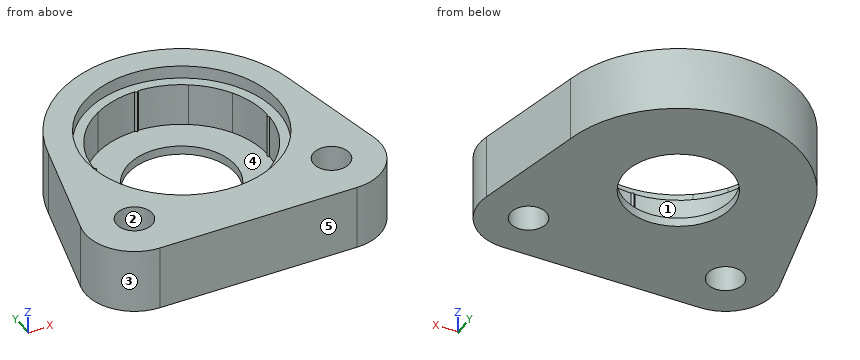
Autodesk Inventor part; units mm, degrees
ref_plane "YZ Plane" through (0, 0, 0) normal (1, 0, 0) x (0, 1, 0)
ref_plane "XZ Plane" through (0, 0, 0) normal (0, 1, 0) x (-1, 0, 0)
ref_plane "XY Plane" through (0, 0, 0) normal (0, 0, 1) x (1, 0, 0)
sketch "Sketch1" plane through (0, 0, 0) normal (0, 0, 1) x (1, 0, 0)
  arc A0 (-5.827627, -9.579088) -> (-0.250527, -11.231057) centre (0.025157, -0.060123) ccw
  arc A1 (0.25, -11.209713) -> (5.829601, -9.582326) centre (0.025157, -0.060123) ccw
  line L0 (0.46552, -11.403002) -> (0, -10.9855)
  line L1 (0, -10.9855) -> (-0.46552, -11.403002)
  arc A2 (-11.176173, -0.249433) -> (-9.579088, -5.827627) centre (0.025157, -0.060123) ccw
  line L2 (-11.403002, -0.46552) -> (-10.9855, 0)
  line L3 (-10.9855, 0) -> (-11.403002, 0.46552)
  arc A3 (-9.579088, 5.827627) -> (-11.209713, 0.25) centre (0, 0) ccw
  arc A4 (5.827627, 9.579088) -> (0.25, 11.209713) centre (0, 0) ccw
  line L4 (0, 10.9855) -> (0.46552, 11.403002)
  line L5 (-0.46552, 11.403002) -> (0, 10.9855)
  arc A5 (-0.25, 11.209713) -> (-5.827627, 9.579088) centre (0, 0) ccw
  arc A6 (11.209713, 0.25) -> (9.579088, 5.827627) centre (0, 0) ccw
  line L6 (11.403002, 0.46552) -> (10.9855, 0)
  line L7 (10.9855, 0) -> (11.403002, -0.46552)
  arc A7 (9.579088, -5.827627) -> (11.209713, -0.25) centre (0, 0) ccw
  arc A8 (7.230816, -10.196338) -> (10.196338, -7.230816) centre (0, 0) ccw
  arc A9 (-10.196338, -7.230816) -> (-7.230816, -10.196338) centre (0, 0) ccw
  arc A10 (-7.230816, 10.196338) -> (-10.196338, 7.230816) centre (0, 0) ccw
  circle A11 centre (0, 0) radius 12.5
  circle A12 centre (12.7, -12.7) radius 2.3241
  circle A13 centre (-12.7, -12.7) radius 2.3241
  line L8 (-19.05, -12.7) -> (19.05, -12.7) construction
  line L9 (-12.7, -19.05) -> (12.7, -19.05)
  line L10 (12.7, -6.35) -> (-12.7, -6.35)
  arc A14 (-12.7, -6.35) -> (-12.7, -19.05) centre (-12.7, -12.7) ccw
  arc A15 (12.7, -19.05) -> (12.7, -6.35) centre (12.7, -12.7) ccw
  circle A16 centre (0, 0) radius 11.2125
  circle A17 centre (0, 0) radius 15.875
  line L11 (15.560093, 3.146287) -> (18.887388, -11.272158)
  line L12 (0, -10.9855) -> (0, -12.5)
  line L13 (-15.560093, 3.146287) -> (-18.887388, -11.272158)
  point P0 (-0.46552, -11.403002)
  point P1 (-11.403002, -0.46552)
  point P2 (0, -12.7)
  point P3 (10.196338, -7.230816)
  point P4 (7.230816, -10.196338)
  point P5 (-7.230816, -10.196338)
  point P6 (-10.196338, -7.230816)
  point P7 (-10.196338, 7.230816)
  point P8 (-7.230816, 10.196338)
  point P9 (-0.25, -11.209713)
  point P10 (0.25, -11.209713)
  point P11 (9.579088, -5.827627)
  point P12 (9.579088, 5.827627)
  point P13 (-5.827627, 9.579088)
  point P14 (-9.579088, 5.827627)
  point P15 (-11.209713, -0.25)
  dimension "d0" = 25
  dimension "d9" = 31.75
  dimension "d1" = 4.6482
  dimension "d2" = 4.6482
  dimension "d4" = 6.35
  dimension "d5" = 6.35
  dimension "d6" = 12.7
  dimension "d8" = 25.4
extrude "Extrusion1" add sketch "Sketch1" along normal blind 12.7 contours L10 A14 A17 A15 A11 A10 | A11 A9 A8 L10 A15 A17 A12 A13 A14 | A17 A13 A12 A15 L9 A14 | A14 L13 A17 | A17 L11 A15
extrude "Extrusion2" add sketch "Sketch1" along normal blind 10.9982 contours A16 L1 A0 | A0 L1 A16 L12 A11 A9 L10 | A16 L10 L0 L1 | A16 L2 L3 A3 A5 L5 L4 A4 A6 L6 L7 A7 L10 | L10 A11 A10 A16 A7 A6 A4 A5 A3 | L1 L12 A16 | L10 A11 A8 L12 A16 | L0 A16 L12 | A16 L3 L2 | L7 L6 A16 | A16 L4 L5
sketch "Sketch1 outline for Extrusion3" plane through (0, 0, 0) normal (0, 0, 1) x (1, 0, 0)
  arc A0 (-11.209713, -0.25) -> (-0.25, -11.209713) centre (0, 0) ccw
  line L0 (-10.9855, 0) -> (-11.209713, -0.25)
  line L1 (-11.209713, 0.25) -> (-10.9855, 0)
  arc A1 (-9.579088, 5.827627) -> (-11.209713, 0.25) centre (0, 0) ccw
  arc A2 (-5.827627, 9.579088) -> (-9.579088, 5.827627) centre (0, 0) ccw
  arc A3 (-0.25, 11.209713) -> (-5.827627, 9.579088) centre (0, 0) ccw
  line L2 (0, 10.9855) -> (-0.25, 11.209713)
  line L3 (0.25, 11.209713) -> (0, 10.9855)
  arc A4 (5.827627, 9.579088) -> (0.25, 11.209713) centre (0, 0) ccw
  arc A5 (9.579088, 5.827627) -> (5.827627, 9.579088) centre (0, 0) ccw
  arc A6 (11.209713, 0.25) -> (9.579088, 5.827627) centre (0, 0) ccw
  line L4 (10.9855, 0) -> (11.209713, 0.25)
  line L5 (11.209713, -0.25) -> (10.9855, 0)
  arc A7 (9.579088, -5.827627) -> (11.209713, -0.25) centre (0, 0) ccw
  arc A8 (0.25, -11.209713) -> (9.579088, -5.827627) centre (0, 0) ccw
  line L6 (0, -10.9855) -> (0.25, -11.209713)
  line L7 (-0.25, -11.209713) -> (0, -10.9855)
extrude "Extrusion3" cut sketch "Sketch1 outline for Extrusion3" along normal blind 10.9982
sketch "Sketch2" plane through (0, 0, 0) normal (0, 0, -1) x (-1, 0, 0)
  arc A0 (-0.25, 11.209713) -> (-11.209713, 0.25) centre (0, 0) ccw
  arc A1 (11.209713, 0.25) -> (0.25, 11.209713) centre (0, 0) ccw
  line L0 (0, 10.9855) -> (0.25, 11.209713)
  line L1 (-0.25, 11.209713) -> (0, 10.9855)
  line L2 (11.209713, 0.25) -> (10.9855, 0)
  line L3 (10.9855, 0) -> (11.209713, -0.25)
  arc A2 (0.25, -11.209713) -> (11.209713, -0.25) centre (0, 0) ccw
  line L4 (0.25, -11.209713) -> (0, -10.9855)
  line L5 (0, -10.9855) -> (-0.25, -11.209713)
  arc A3 (-11.209713, -0.25) -> (-0.25, -11.209713) centre (0, 0) ccw
  line L6 (-11.209713, -0.25) -> (-10.9855, 0)
  line L7 (-10.9855, 0) -> (-11.209713, 0.25)
  circle A4 centre (0, 0) radius 6.9977
  point P0 (0, 0)
  dimension "d16" = 13.9954
extrude "Extrusion4" add sketch "Sketch2" against normal blind 5.3848
sketch "Sketch3" plane through (0, 0, 0) normal (0, 0, -1) x (-1, 0, 0)
  circle A0 centre (0, 0) radius 6.9977
  arc A1 (12.7, -19.05) -> (18.887388, -11.272158) centre (12.7, -12.7) ccw
  line L0 (15.560093, 3.146287) -> (18.887388, -11.272158)
  arc A2 (15.560093, 3.146287) -> (-15.560093, 3.146287) centre (0, 0) ccw
  line L1 (-18.887388, -11.272158) -> (-15.560093, 3.146287)
  arc A3 (-18.887388, -11.272158) -> (-12.7, -19.05) centre (-12.7, -12.7) ccw
  line L2 (12.7, -19.05) -> (-12.7, -19.05)
  circle A4 centre (12.7, -12.7) radius 2.3241
  circle A5 centre (-12.7, -12.7) radius 2.3241
  point P0 (0, 0)
extrude "Extrusion5" cut sketch "Sketch3" against normal blind 4.233333
sketch "Sketch4" plane through (0, 0, 4.233333) normal (0, 0, -1) x (-1, 0, 0)
  point P0 (0, 0)
sketch "Sketch5" plane through (0, 0, 4.233333) normal (0, 0, -1) x (-1, 0, 0)
  point P0 (0, 0)
properties part number "Conveyor Bearing Housing"
Verification items for the finished model (mm, model axes). Face numbers are marked on the shaded views. A direction names the side the tool comes from. Coordinates: 2 decimals unless noted, no trailing zeros. Write each loop counter-clockwise with the first axis right and the second up, starting at its lowest first coordinate (ties: lowest second). Pieces come first, ordered by that corner, then holes. Notation, with made-up numbers: M 5.5,72 L 55.5,72 A24 cw 55.5,106 Z; hole C 62.25,47.25 d5. An arc over 180 degrees is marked long. Use a Markdown table: item, result.
Q1. Set-up check for the marked faces 1 and 2: record each of +Z, -Z, +X, -X, +Y, -Y from which the full face is reachable in a straight line by a thin tool's end or side.
Reply:
| item | result |
|---|---|
| face 1 | +Z |
| face 2 | +Z, -Z |
Q2. Go/stop test with flat-tipped pins: P1, Ø1, axis at y = -9.5, z = 11.5, coming from the +X side; P2, Ø12.5, axis at x = -3.5, y = 1.5, coming from the +Z side; P3, Ø1, axis at y = -8, z = 6, coming from the +X side. Record where each tip stops, or that it passes through.
Reply:
| item | result |
|---|---|
| P1 | stops at x = 18.59 |
| P2 | stops at z = 5.38 |
| P3 | stops at x = 18.25 |
Q3. Draft check along X on the marked faces 3, 4 and 5. Enter one of: +X half, -X half, draft (parallel to the pull), parting line (faces both ways), or undercut.
Reply:
| item | result |
|---|---|
| face 3 | -X half |
| face 4 | undercut |
| face 5 | draft |
Q4. Sectioned sample at C-C, the plane y = 10. Record the boundary of the cut face in (x, z), plus the area to 3 significant figures.
Reply:
| item | result |
|---|---|
| outline | M -12.33,4.23 L 12.33,4.23 L 12.33,12.7 L 7.5,12.7 L 7.5,11 L 5.07,11 L 5.07,5.38 L -5.07,5.38 L -5.07,11 L -7.5,11 L -7.5,12.7 L -12.33,12.7 Z |
| area | 126 mm² |
Q5. Sectioned sample at B-B, the plane x = -12. Record the boundary of the cut face in (y, z).
Reply:
| item | result |
|---|---|
| outline | M -19.05,4.23 L -14.92,4.23 L -14.92,12.7 L -19.05,12.7 Z; M -10.48,4.23 L 10.39,4.23 L 10.39,12.7 L 3.5,12.7 L 3.5,11 L -3.5,11 L -3.5,12.7 L -10.48,12.7 Z |
Q6. Sectioned sample at A-A, the plane z = 6.5. Count the separate pieces of the cut face and the enclosed holes in it, plus the area to 3 significant figures.
Reply:
| item | result |
|---|---|
| separate pieces | 1 |
| enclosed holes | 3 |
| area | 644 mm² |
Q7. Thickness scan on line 1 (X direction, y = -12.7, z = 9.5); line 2 (Y direction, x = 0, z = 5.1) (3 decimals); line 3 (Y direction, x = -11.5, z = 8.5). Record the ranges inside material, lowest first.
Reply:
| item | result |
|---|---|
| line 1 | x = -19.05 to -15.02, -10.38 to 10.38, 15.02 to 19.05 |
| line 2 | y = -19.05 to -6.998, 6.998 to 15.875 |
| line 3 | y = -19.05 to -14.69, -10.71 to 10.94 |
Q8. Sectioned sample at D-D, the plane x = 16. Record the boundary of the cut face in (y, z).
Reply:
| item | result |
|---|---|
| outline | M -18.13,4.23 L 1.24,4.23 L 1.24,12.7 L -18.13,12.7 Z |
